Check sheet for the modelled part. Datum: model origin and axes. Units: mm. Round coordinates to 2 decimals unless told otherwise and drop trailing zeros. Write each loop counter-clockwise with the first axis right and the second up, starting at its lowest first coordinate (ties: lowest second). Pieces come first, ordered by that corner, then holes. Notation, with made-up numbers: (69, -23.5) -> (96, -23.5) arc R26 cw to (96, 15.5) -> close; hole circle Ø9 at (52.5, 14). An arc over 180 degrees is marked (long way). One line per item, written item: value.
from build123d import *

# Parameters (mm, degrees)
SKETCH1_R           = 3.3
BOSS_EXTRUDE3_DEPTH = 2.54
FILLET1_R           = 2.54
FILLET2_R           = 2.54


with BuildPart() as part:
    # Sketch1 → Boss-Extrude3 (new body)
    with BuildSketch(Plane.XY):
        with BuildLine():
            Line((24.307803938, -29.663229905), (-6.055469212, -11.163390731))
            Line((-6.055469212, -11.163390731), (8.577809795, 9.365424663))
            Line((8.577809795, 9.365424663), (35.556707766, -14.378954182))
            ThreePointArc((35.556707766, -14.378954182), (36.935104815, -27.175040842), (24.307803938, -29.663229905))
        make_face()
        with Locations((29.263786665, -21.529112854)):
            Circle(SKETCH1_R, mode=Mode.SUBTRACT)
    extrude(amount=BOSS_EXTRUDE3_DEPTH)

    # Fillet1
    fillet1_edges = [part.edges().sort_by_distance(p)[0] for p in [
        (-6.055469212, -11.163390731, 1.27),
    ]]
    fillet(fillet1_edges, radius=FILLET1_R)

    # Fillet2
    fillet2_edges = [part.edges().sort_by_distance(p)[0] for p in [
        (8.577809795, 9.365424663, 1.27),
    ]]
    fillet(fillet2_edges, radius=FILLET2_R)


solid = part.part
Item 1: Mould release check, pull along Y, two halves, no side actions. Record for faces 1 (the flat face through (1.157, -1.046, 1.252)), 2 (the flat face through (10.488, -21.243, 1.252)), 3 (the cylindrical face through (32.312, -22.793, 1.252)), 4 (the cylindrical face through (37.051, -27.015, 1.252)): pulls with the +Y half, pulls with the -Y half, needs draft (parallel to the pull), parting line crosses it, or undercut.
Answer:
face 1: pulls with the +Y half
face 2: pulls with the -Y half
face 3: undercut
face 4: parting line crosses it
Item 2: Sectioned sample at C-C on x = 1. Enter the section's corners in (y, z), and give its area (3 significant figures).
Answer:
outline: (-15.46, 0) -> (-1.27, 0) -> (-1.27, 2.54) -> (-15.46, 2.54) -> close
area: 36.1 mm^2
Item 3: Thickness scan on line 1 (Y direction, x = 27.5, z = 0.95); line 2 (X direction, y = -20, z = 0.4); line 3 (X direction, y = -19, z = 2.35). Record the ranges inside material, lowest first.
Answer:
line 1: y = -30.89 to -24.32, -18.74 to -7.29
line 2: x = 8.45 to 26.34, 32.19 to 38.67
line 3: x = 6.81 to 27.14, 31.38 to 38.45
Item 4: Sectioned sample at A-A on z = 1.4. Enter the section's corners in (x, y) (3 decimals), and give its area (3 significant figures).
Answer:
outline: (-4.471, -8.94) arc R2.54 ccw to (-3.724, -12.584) -> (24.308, -29.663) arc R9.525 ccw to (35.557, -14.379) -> (10.691, 7.506) arc R2.54 ccw to (6.944, 7.074) -> close; hole circle Ø6.6 at (29.264, -21.529)
area: 876 mm^2
Item 5: Sectioned sample at B-B on y = -1.5. Enter the section's corners in (x, z).
Answer:
outline: (0.83, 0) -> (20.92, 0) -> (20.92, 2.54) -> (0.83, 2.54) -> close
